The listing builds one solid part. Answer for the finished solid, in the listing's coordinates (mm). A direction names the side the tool comes from. Coordinates: 2 decimals unless noted, no trailing zeros. Loops run counter-clockwise (first coordinate to the right, second up) from the corner with the lowest first, then second, coordinate; pieces in that order, holes last. Notation, with made-up numbers: (75, -3.75) -> (102, -3.75) arc R17 ccw to (102, 5.25) -> close; hole circle Ø1 at (21.25, -3.5). An arc over 180 degrees is marked (long way). Answer in a Markdown table with one row per item.
```python
from build123d import *

# Parameters (mm, degrees)
SKETCH3_R           = 20
SKETCH3_R_2         = 5
SKETCH6_R           = 20
SKETCH6_R_2         = 5
BOSS_EXTRUDE1_DEPTH = 8
SKETCH10_W          = 6
SKETCH10_H          = 6
CUT_EXTRUDE5_DEPTH  = 5


with BuildPart() as part:
    # Sweep1: sweep along a path in Sketch2
    with BuildLine(Plane(origin=(0, 0, 0), x_dir=(0, 0, -1), z_dir=(1, 0, 0))) as sweep1_path:
        ThreePointArc((30, 0), (21.213203436, 21.213203436), (0, 30))
    # Sketch3 → Sweep1 (sweep)
    with BuildSketch(Plane(origin=(0, 0, 0), x_dir=(1, 0, 0), z_dir=(0, 1, 0))):
        with Locations((0, 30)):
            Circle(SKETCH3_R)
        with Locations((0, 30)):
            Circle(SKETCH3_R_2, mode=Mode.SUBTRACT)
    sweep(path=sweep1_path.line)

    # Sketch6 → Boss-Extrude1 (add)
    with BuildSketch(Plane.XZ):
        with Locations((0, -30)):
            Circle(SKETCH6_R)
        with Locations((0, -30)):
            Circle(SKETCH6_R_2, mode=Mode.SUBTRACT)
    extrude(amount=BOSS_EXTRUDE1_DEPTH)

    # Sketch10 → Cut-Extrude5 (cut)
    with BuildSketch(Plane.XY):
        with Locations((0, 42.5)):
            Rectangle(SKETCH10_W, SKETCH10_H)
        with Locations((-12.5, 30)):
            Rectangle(SKETCH10_W, SKETCH10_H)
        with Locations((12.5, 30)):
            Rectangle(SKETCH10_W, SKETCH10_H)
        with Locations((0, 17.5)):
            Rectangle(SKETCH10_W, SKETCH10_H)
    extrude(amount=-CUT_EXTRUDE5_DEPTH, mode=Mode.SUBTRACT)


solid = part.part
```
Item 1: Determine the mould class of faces 4 (the face through (4, 34, 0)), 5 (the face through (0, 18, -5)) for opening direction X: +X half, -X half, draft (parallel to the pull), parting line (faces both ways), or undercut.
Findings below:
| item | result |
|---|---|
| face 4 | draft |
| face 5 | undercut |
Item 2: Flat-ended cylindrical pins translate along their axes: pin 1 Ø1 at (x, z) = (-7.5, -43) entering from +Y; pin 2 Ø5.5 at (x, z) = (-1.5, -1.5) entering from +Y; pin 3 Ø5 at (x, y) = (-15.5, 31) entering from -Z. Find the tip coordinate at first contact, or state that the pin passes through.
Findings below:
| item | result |
|---|---|
| pin 1 | stops at y = 23.54 |
| pin 2 | stops at y = 50 |
| pin 3 | stops at z = -33.66 |
Item 3: A tool of negligible diameter and unlimited length cuts with its end or side. For faces 1 (the face through (-3, 42, -2)), 2 (the face through (4, -8, -34)), 3 (the face through (-1.08, -3.94, -34.88)), from which of +Z, -Z, +X, -X, +Y, -Y can it reach the whole face along a straight path? Write none if from no direction.
Findings below:
| item | result |
|---|---|
| face 1 | +Z |
| face 2 | +Z, -Z, +X, -X, -Y |
| face 3 | -Y |
Item 4: A cutting plane is placed at A-A, the plane x = 0. Determine the outline of the cut face in (y, z).
Findings below:
| item | result |
|---|---|
| outline | (-8, -50) -> (0, -50) arc R50 ccw to (50, 0) -> (45.5, 0) -> (45.5, -5) -> (39.5, -5) -> (39.5, 0) -> (35, 0) arc R35 cw to (0, -35) -> (-8, -35) -> close; (-8, -25) -> (0, -25) arc R25 ccw to (25, 0) -> (20.5, 0) -> (20.5, -5) -> (14.5, -5) -> (14.5, 0) -> (10, 0) arc R10 cw to (0, -10) -> (-8, -10) -> close |
Item 5: Find the intervals of material crossed by probe 1 along Z at (x, y) = (0, -5); probe 2 along Y at (x, z) = (1, -30); probe 3 along Y at (x, z) = (14, -6), in increasing order.
Findings below:
| item | result |
|---|---|
| probe 1 | z = -50 to -35, -25 to -10 |
| probe 2 | y = 17.83 to 39.97 |
| probe 3 | y = 14.53 to 43.87 |
